Read the model definition and answer for the solid it produces. Units are mm, in the model's axes. A direction names the side the tool comes from. Give positions to 0.01 mm unless a question says otherwise; leave off trailing zeros. Write each loop counter-clockwise with the first axis right and the second up, starting at its lowest first coordinate (ties: lowest second). Pieces come first, ordered by that corner, then holes. Notation, with made-up numbers: (63.25, 16) -> (102.25, 16) arc R29 cw to (102.25, 41) -> close; hole circle Ø1 at (67.5, 2). An arc over 180 degrees is marked (long way). Answer as CSV lines item,"result". Start each with the question number.
1. The part is cut by section C-C, the plane y = -8. Determine the outline of the cut face in (x, z), and give its area (3 significant figures).
2. The part is cut by section B-B, the plane y = 10.5. Determine the outline of the cut face in (x, z), and give its area (3 significant figures).
3. A tool of negligible diameter and unlimited length cuts with its end or side. For faces 1 (the cylindrical face through (-3.909, -17.605, 2.576)), 2 (the flat face through (-3, 18, 3.81)), from which of +Z, -Z, +X, -X, +Y, -Y can it reach the whole face along a straight path? Write none if from no direction.
4. Given pin 1 (1 mm diameter, centred on x = 13.5, z = 3.5, fed in from +Y); pin 2 (0.8 mm diameter, centred on y = 6.5, z = 2, fed in from +X); pin 3 (2 mm diameter, centred on y = 16.5, z = 2, fed in from -X), each flat-ended and moving along its own axis, determine where each tip first touches the part or whether it passes through.
5. Find the intervals of material crossed by line 1 (Y direction, x = 0, z = 3.85); line 2 (Y direction, x = 0, z = 2.75), in increasing order.
6. For a pull along Z with two mould halves and no side action, classify faces 3 (the flat face through (-13, -13, 0)), 4 (the flat face through (-13, -13, 5.08)), 5 (the flat face through (-18.034, 6, 3)), 6 (the flat face through (18.034, 6, 3)) as pulls with the +Z half, pulls with the -Z half, needs draft (parallel to the pull), parting line crosses it, or undercut.
7. The part is cut by section A-A, the plane x = 0. Determine the outline of the cut face in (y, z).
8. The part is cut by section D-D, the plane z = 2.05. Determine the outline of the cut face in (x, y).
from build123d import *
from build123d.topology import SkipClean

# Parameters (mm, degrees)
SKETCH1_R                = 21.59
BOSS_EXTRUDE1_DEPTH      = 5.08
SKETCH4_R                = 18.034
CUT_EXTRUDE1_DEPTH       = 31.952586322
SKETCH5_W                = 43.18
SKETCH5_H                = 2.54
CUT_EXTRUDE2_DEPTH       = 31.952586322
BOSS_EXTRUDE2_REACH      = 32.953
BOSS_EXTRUDE2_END_RADIUS = 21.59
SKETCH6_W                = 3.556
SKETCH6_H                = 2.54


with BuildPart() as part:
    # Sketch1 → Boss-Extrude1 (new body)
    with BuildSketch(Plane.XY):
        Circle(SKETCH1_R)
    extrude(amount=BOSS_EXTRUDE1_DEPTH)

    # Sketch4 → Cut-Extrude1 (cut, through all)
    with BuildSketch(Plane.XY.offset(5.08)):
        Circle(SKETCH4_R)
    extrude(amount=-CUT_EXTRUDE1_DEPTH, mode=Mode.SUBTRACT)

    # Sketch5 → Cut-Extrude2 (cut, through all)
    with BuildSketch(Plane(origin=(0, 0, 0), x_dir=(1, 0, 0), z_dir=(0, 1, 0))):
        with Locations((0, -2.54)):
            Rectangle(SKETCH5_W, SKETCH5_H)
    extrude(amount=CUT_EXTRUDE2_DEPTH, mode=Mode.SUBTRACT)

    # Boss-Extrude2: up to this cylinder (the profile starts inside it)
    with SkipClean():  # the faces are left unmerged after this step: merging them gives an invalid solid
        boss_extrude2_end = Plane(origin=(0, 0, 2.54), z_dir=(0, 0, -1)) * Cylinder(BOSS_EXTRUDE2_END_RADIUS, 110.086, mode=Mode.PRIVATE)
        # Sketch6 → Boss-Extrude2 (add, up to the surface)
        with BuildSketch(Plane(origin=(0, 0, 0), x_dir=(1, 0, 0), z_dir=(0, 1, 0)), mode=Mode.PRIVATE) as boss_extrude2_sk1:
            with Locations((-19.812, -2.54)):
                Rectangle(SKETCH6_W, SKETCH6_H)
        boss_extrude2_tool1 = extrude(boss_extrude2_sk1.sketch, amount=BOSS_EXTRUDE2_REACH, mode=Mode.PRIVATE) & boss_extrude2_end
        add(boss_extrude2_tool1.solids().sort_by_distance((-19.812, 0, 2.54))[0])
        # Sketch6 → Boss-Extrude2 (add, up to the surface)
        with BuildSketch(Plane(origin=(0, 0, 0), x_dir=(1, 0, 0), z_dir=(0, 1, 0)), mode=Mode.PRIVATE) as boss_extrude2_sk2:
            with Locations((19.812, -2.54)):
                Rectangle(SKETCH6_W, SKETCH6_H)
        boss_extrude2_tool2 = extrude(boss_extrude2_sk2.sketch, amount=BOSS_EXTRUDE2_REACH, mode=Mode.PRIVATE) & boss_extrude2_end
        add(boss_extrude2_tool2.solids().sort_by_distance((19.812, 0, 2.54))[0])


solid = part.part
Results found:
1,outline,"(-20.05, 0) -> (-16.16, 0) -> (-16.16, 5.08) -> (-20.05, 5.08) -> close; (16.16, 0) -> (20.05, 0) -> (20.05, 5.08) -> (16.16, 5.08) -> close"
1,area,"39.5 mm²"
2,outline,"(-18.86, 0) -> (-14.66, 0) -> (-14.66, 1.27) -> (-18.03, 1.27) -> (-18.03, 3.81) -> (-14.66, 3.81) -> (-14.66, 5.08) -> (-18.86, 5.08) -> close; (14.66, 0) -> (18.86, 0) -> (18.86, 5.08) -> (14.66, 5.08) -> (14.66, 3.81) -> (18.03, 3.81) -> (18.03, 1.27) -> (14.66, 1.27) -> close"
2,area,"25.6 mm²"
3,face 1,"+Z, -Z"
3,face 2,"+Y"
4,pin 1,"stops at y = 17.16"
4,pin 2,"stops at x = 20.71"
4,pin 3,"stops at x = -14.7"
5,line 1,"y = -21.59 to -18.03, 18.03 to 21.59"
5,line 2,"y = -21.59 to -18.03"
6,face 3,"pulls with the -Z half"
6,face 4,"pulls with the +Z half"
6,face 5,"undercut"
6,face 6,"undercut"
7,outline,"(-21.59, 0) -> (-18.03, 0) -> (-18.03, 5.08) -> (-21.59, 5.08) -> close; (18.03, 0) -> (21.59, 0) -> (21.59, 1.27) -> (18.03, 1.27) -> close; (18.03, 3.81) -> (21.59, 3.81) -> (21.59, 5.08) -> (18.03, 5.08) -> close"
8,outline,"(-18.03, 0) -> (-18.03, 11.87) arc R21.59 ccw (long way) to (18.03, 11.87) -> (18.03, 0) arc R18.03 cw to start"
